Geometry: final body of the model. Coordinates: model frame, mm. Give positions to 0.01 mm unless a question says otherwise; leave off trailing zeros. Loops run counter-clockwise (first coordinate to the right, second up) from the corner with the lowest first, then second, coordinate; pieces in that order, holes last.
from build123d import *

# Parameters (mm, degrees)
SKETCH1_R           = 1.5875
BOSS_EXTRUDE5_DEPTH = 1.5875
FILLET2_R           = 2.54
FILLET3_R           = 2.54
FILLET4_R           = 5.08
CUT_EXTRUDE1_START  = -2.54
SKETCH2_R           = 2.38125
SKETCH2_R_2         = 1.5875
CUT_EXTRUDE1_DEPTH  = 2.54
SKETCH3_R           = 1.5875
CUT_EXTRUDE2_DEPTH  = 2.54
CUT_EXTRUDE3_DEPTH  = 2.54
SKETCH5_W           = 15
SKETCH5_H           = 34.925
CUT_EXTRUDE4_DEPTH  = 109.650407999
FILLET5_R           = 7.62
FILLET6_R           = 7.62
SKETCH6_R           = 79.375
CUT_EXTRUDE5_DEPTH  = 0.5875


with BuildPart() as part:
    # Sketch1 → Boss-Extrude5 (new body)
    with BuildSketch(Plane(origin=(0, 0, 0), x_dir=(1, 0, 0), z_dir=(0, 1, 0))):
        with BuildLine():
            ThreePointArc((-63.5, -47.625), (-35.497579143, -70.995158286), (0, -79.375))
            ThreePointArc((0, -79.375), (35.497579143, -70.995158286), (63.5, -47.625))
            Line((63.5, -47.625), (50.8, -47.625))
            Line((50.8, -47.625), (50.8, 22.225))
            Line((50.8, 22.225), (76.2, 22.225))
            ThreePointArc((76.2, 22.225), (0, 79.375), (-76.2, 22.225))
            Line((-76.2, 22.225), (-50.8, 22.225))
            Line((-50.8, 22.225), (-50.8, -47.625))
            Line((-50.8, -47.625), (-63.5, -47.625))
        make_face()
        with Locations(Location((-7.14375, -66.675, 0), (0, 0, 270))):
            Circle(SKETCH1_R, mode=Mode.SUBTRACT)
        with BuildLine():
            ThreePointArc((8.73125, -66.675), (7.14375, -68.2625), (5.55625, -66.675))
            ThreePointArc((5.55625, -66.675), (7.14375, -65.0875), (8.73125, -66.675))
        make_face(mode=Mode.SUBTRACT)
        with Locations(Location((-7.14375, 66.675, 0), (0, 0, 270))):
            Circle(SKETCH1_R, mode=Mode.SUBTRACT)
        with Locations(Location((7.14375, 66.675, 0), (0, 0, 270))):
            Circle(SKETCH1_R, mode=Mode.SUBTRACT)
    extrude(amount=BOSS_EXTRUDE5_DEPTH)

    # Fillet2
    fillet2_edges = [part.edges().sort_by_distance(p)[0] for p in [
        (-63.5, 0.79375, 47.625),
    ]]
    fillet(fillet2_edges, radius=FILLET2_R)

    # Fillet3
    fillet3_edges = [part.edges().sort_by_distance(p)[0] for p in [
        (63.5, 0.79375, 47.625),
    ]]
    fillet(fillet3_edges, radius=FILLET3_R)

    # Fillet4
    fillet4_edges = [part.edges().sort_by_distance(p)[0] for p in [
        (-76.2, 0.79375, -22.225),
        (76.2, 0.79375, -22.225),
    ]]
    fillet(fillet4_edges, radius=FILLET4_R)

    # Sketch2 → Cut-Extrude1 (cut)
    # profile 1 of 10: a face of its own
    with BuildSketch(Plane(origin=(0, 1.5875, 0), x_dir=(1, 0, 0), z_dir=(0, 1, 0)).offset(CUT_EXTRUDE1_START)):
        with BuildLine():
            Line((-61.088622125, 27.654457796), (-59.642408406, 26.999765402))
            ThreePointArc((-59.642408406, 26.999765402), (-52.384826382, 39.268743005), (-42.643785254, 49.676068599))
            Line((-42.643785254, 49.676068599), (-43.677815048, 50.880617741))
            Line((-43.677815048, 50.880617741), (-44.711844841, 52.085166883))
            ThreePointArc((-44.711844841, 52.085166883), (-54.925289002, 41.173126022), (-62.534835843, 28.309150189))
            Line((-62.534835843, 28.309150189), (-61.088622125, 27.654457796))
        make_face()
    # profile 2 of 10: a face of its own
    with BuildSketch(Plane(origin=(0, 1.5875, 0), x_dir=(1, 0, 0), z_dir=(0, 1, 0)).offset(CUT_EXTRUDE1_START)):
        with BuildLine():
            Line((-39.077069744, 54.493774041), (-38.151958122, 53.203686937))
            ThreePointArc((-38.151958122, 53.203686937), (-25.732218917, 60.200142208), (-12.092567045, 64.342629994))
            Line((-12.092567045, 64.342629994), (-12.385788543, 65.902815048))
            Line((-12.385788543, 65.902815048), (-12.679010041, 67.463000102))
            ThreePointArc((-12.679010041, 67.463000102), (-26.980132574, 63.119617589), (-40.002181367, 55.783861145))
            Line((-40.002181367, 55.783861145), (-39.077069744, 54.493774041))
        make_face()
    # profile 3 of 10: a face of its own
    with BuildSketch(Plane(origin=(0, 1.5875, 0), x_dir=(1, 0, 0), z_dir=(0, 1, 0)).offset(CUT_EXTRUDE1_START)):
        with Locations(Location((-7.14375, 66.675, 0), (0, 0, 270))):
            Circle(SKETCH2_R)
        with Locations((-7.14375, 66.675)):
            Circle(SKETCH2_R_2, mode=Mode.SUBTRACT)
    # profile 4 of 10: a face of its own
    with BuildSketch(Plane(origin=(0, 1.5875, 0), x_dir=(1, 0, 0), z_dir=(0, 1, 0)).offset(CUT_EXTRUDE1_START)):
        with Locations(Location((7.14375, 66.675, 0), (0, 0, 270))):
            Circle(SKETCH2_R)
        with Locations((7.14375, 66.675)):
            Circle(SKETCH2_R_2, mode=Mode.SUBTRACT)
    # profile 5 of 10: a face of its own
    with BuildSketch(Plane(origin=(0, 1.5875, 0), x_dir=(1, 0, 0), z_dir=(0, 1, 0)).offset(CUT_EXTRUDE1_START)):
        with BuildLine():
            ThreePointArc((12.679010041, 67.463000102), (26.980132574, 63.119617589), (40.002181367, 55.783861145))
            Line((40.002181367, 55.783861145), (39.077069744, 54.493774041))
            Line((39.077069744, 54.493774041), (38.151958122, 53.203686937))
            ThreePointArc((38.151958122, 53.203686937), (25.732218917, 60.200142208), (12.092567045, 64.342629994))
            Line((12.092567045, 64.342629994), (12.385788543, 65.902815048))
            Line((12.385788543, 65.902815048), (12.679010041, 67.463000102))
        make_face()
    # profile 6 of 10: a face of its own
    with BuildSketch(Plane(origin=(0, 1.5875, 0), x_dir=(1, 0, 0), z_dir=(0, 1, 0)).offset(CUT_EXTRUDE1_START)):
        with BuildLine():
            ThreePointArc((44.711844841, 52.085166883), (54.925289002, 41.173126022), (62.534835843, 28.309150189))
            Line((62.534835843, 28.309150189), (59.642408406, 26.999765402))
            ThreePointArc((59.642408406, 26.999765402), (52.384826382, 39.268743005), (42.643785254, 49.676068599))
            Line((42.643785254, 49.676068599), (43.677815048, 50.880617741))
            Line((43.677815048, 50.880617741), (44.711844841, 52.085166883))
        make_face()
    # profile 7 of 10: a face of its own
    with BuildSketch(Plane(origin=(0, 1.5875, 0), x_dir=(1, 0, 0), z_dir=(0, 1, 0)).offset(CUT_EXTRUDE1_START)):
        with BuildLine():
            ThreePointArc((-12.679010041, -67.463000102), (-26.980132574, -63.119617589), (-40.002181367, -55.783861145))
            Line((-40.002181367, -55.783861145), (-39.077069744, -54.493774041))
            Line((-39.077069744, -54.493774041), (-38.151958122, -53.203686937))
            ThreePointArc((-38.151958122, -53.203686937), (-25.732218917, -60.200142208), (-12.092567045, -64.342629994))
            Line((-12.092567045, -64.342629994), (-12.385788543, -65.902815048))
            Line((-12.385788543, -65.902815048), (-12.679010041, -67.463000102))
        make_face()
    # profile 8 of 10: a face of its own
    with BuildSketch(Plane(origin=(0, 1.5875, 0), x_dir=(1, 0, 0), z_dir=(0, 1, 0)).offset(CUT_EXTRUDE1_START)):
        with Locations(Location((-7.14375, -66.675, 0), (0, 0, 270))):
            Circle(SKETCH2_R)
        with Locations((-7.14375, -66.675)):
            Circle(SKETCH2_R_2, mode=Mode.SUBTRACT)
    # profile 9 of 10: a face of its own
    with BuildSketch(Plane(origin=(0, 1.5875, 0), x_dir=(1, 0, 0), z_dir=(0, 1, 0)).offset(CUT_EXTRUDE1_START)):
        with Locations(Location((7.14375, -66.675, 0), (0, 0, 270))):
            Circle(SKETCH2_R)
        with Locations((7.14375, -66.675)):
            Circle(SKETCH2_R_2, mode=Mode.SUBTRACT)
    # profile 10 of 10: a face of its own
    with BuildSketch(Plane(origin=(0, 1.5875, 0), x_dir=(1, 0, 0), z_dir=(0, 1, 0)).offset(CUT_EXTRUDE1_START)):
        with BuildLine():
            ThreePointArc((12.092567045, -64.342629994), (25.732218917, -60.200142208), (38.151958122, -53.203686937))
            Line((38.151958122, -53.203686937), (39.077069744, -54.493774041))
            Line((39.077069744, -54.493774041), (40.002181367, -55.783861145))
            ThreePointArc((40.002181367, -55.783861145), (26.980132574, -63.119617589), (12.679010041, -67.463000102))
            Line((12.679010041, -67.463000102), (12.385788543, -65.902815048))
            Line((12.385788543, -65.902815048), (12.092567045, -64.342629994))
        make_face()
    extrude(amount=CUT_EXTRUDE1_DEPTH, mode=Mode.SUBTRACT)

    # Sketch3 → Cut-Extrude2 (cut)
    with BuildSketch(Plane(origin=(0, 1.5875, 0), x_dir=(1, 0, 0), z_dir=(0, 1, 0))):
        with Locations(Location((-44.45, -47.625, 0), (0, 0, 270))):
            Circle(SKETCH3_R)
        with Locations(Location((-44.45, 22.225, 0), (0, 0, 270))):
            Circle(SKETCH3_R)
        with Locations(Location((44.45, 22.225, 0), (0, 0, 270))):
            Circle(SKETCH3_R)
        with Locations(Location((44.45, -47.625, 0), (0, 0, 270))):
            Circle(SKETCH3_R)
    extrude(amount=-CUT_EXTRUDE2_DEPTH, mode=Mode.SUBTRACT)

    # Sketch4 → Cut-Extrude3 (cut)
    with BuildSketch(Plane(origin=(0, 1.5875, 0), x_dir=(1, 0, 0), z_dir=(0, 1, 0))):
        with BuildLine():
            ThreePointArc((-44.45, -11.1125), (-46.0375, -12.7), (-44.45, -14.2875))
            Line((-44.45, -14.2875), (-44.45, -11.1125))
        make_face()
        with BuildLine():
            Line((-44.45, -11.1125), (-44.45, -14.2875))
            ThreePointArc((-44.45, -14.2875), (-43.327467985, -13.822532015), (-42.8625, -12.7))
            ThreePointArc((-42.8625, -12.7), (-43.327467985, -11.577467985), (-44.45, -11.1125))
        make_face()
        with BuildLine():
            ThreePointArc((44.45, -11.1125), (42.8625, -12.7), (44.45, -14.2875))
            Line((44.45, -14.2875), (44.45, -11.1125))
        make_face()
        with BuildLine():
            Line((44.45, -11.1125), (44.45, -14.2875))
            ThreePointArc((44.45, -14.2875), (45.572532015, -13.822532015), (46.0375, -12.7))
            ThreePointArc((46.0375, -12.7), (45.572532015, -11.577467985), (44.45, -11.1125))
        make_face()
    extrude(amount=-CUT_EXTRUDE3_DEPTH, mode=Mode.SUBTRACT)

    # Sketch5 → Cut-Extrude4 (cut, through all)
    with BuildSketch(Plane(origin=(0, 1.5875, 0), x_dir=(1, 0, 0), z_dir=(0, 1, 0))):
        with Locations((-27.3, 4.7625)):
            Rectangle(SKETCH5_W, SKETCH5_H)
        with Locations((27.3, 4.7625)):
            Rectangle(SKETCH5_W, SKETCH5_H)
    extrude(amount=-CUT_EXTRUDE4_DEPTH, mode=Mode.SUBTRACT)

    # Fillet5
    # the kernel refuses this fillet: 7.62 mm, written as the material it adds along each edge
    with BuildSketch(Plane(origin=(-19.8, 1.5875, 12.7), x_dir=(0, 0, -1), z_dir=(0, -1, 0))) as fillet5_piece_1:
        with BuildLine():
            CenterArc((FILLET5_R, -FILLET5_R), FILLET5_R, 90, 90)
            Line((0, -FILLET5_R), (0, 0))
            Line((0, 0), (FILLET5_R, 0))
        make_face()
    extrude(amount=1.5875)
    with BuildSketch(Plane(origin=(-34.8, 1.5875, 12.7), x_dir=(0, 0, -1), z_dir=(0, -1, 0)), Plane(origin=(-19.8, 1.5875, -22.225), x_dir=(0, 0, 1), z_dir=(0, -1, 0)), Plane(origin=(-34.8, 1.5875, -22.225), x_dir=(1, 0, 0), z_dir=(0, -1, 0))) as fillet5_piece_2:
        with BuildLine():
            CenterArc((FILLET5_R, FILLET5_R), FILLET5_R, 180, 90)
            Line((0, FILLET5_R), (0, 0))
            Line((0, 0), (FILLET5_R, 0))
        make_face()
    extrude(amount=1.5875)

    # Fillet6
    # the kernel refuses this fillet: 7.62 mm, written as the material it adds along each edge
    with BuildSketch(Plane(origin=(34.8, 1.5875, 12.7), x_dir=(0, 0, -1), z_dir=(0, -1, 0)), Plane(origin=(34.8, 1.5875, -22.225), x_dir=(-1, 0, 0), z_dir=(0, -1, 0))) as fillet6_piece_1:
        with BuildLine():
            CenterArc((FILLET6_R, -FILLET6_R), FILLET6_R, 90, 90)
            Line((0, -FILLET6_R), (0, 0))
            Line((0, 0), (FILLET6_R, 0))
        make_face()
    extrude(amount=1.5875)
    with BuildSketch(Plane(origin=(19.8, 1.5875, -22.225), x_dir=(1, 0, 0), z_dir=(0, -1, 0)), Plane(origin=(19.8, 1.5875, 12.7), x_dir=(0, 0, -1), z_dir=(0, -1, 0))) as fillet6_piece_2:
        with BuildLine():
            CenterArc((FILLET6_R, FILLET6_R), FILLET6_R, 180, 90)
            Line((0, FILLET6_R), (0, 0))
            Line((0, 0), (FILLET6_R, 0))
        make_face()
    extrude(amount=1.5875)

    # Sketch6 → Cut-Extrude5 (cut)
    with BuildSketch(Plane(origin=(0, 0, 0), x_dir=(-1, 0, 0), z_dir=(0, -1, 0))):
        Circle(SKETCH6_R)
    extrude(amount=-CUT_EXTRUDE5_DEPTH, mode=Mode.SUBTRACT)


solid = part.part
Item 1: Section query C-C on z = 32. Return loops of the section in (x, y).
Values follow:
outline: (-50.8, 0.59) - (50.8, 0.59) - (50.8, 1.59) - (-50.8, 1.59) - close
Item 2: Pin query (flat end, axial travel): pin 1 (0.5 mm diameter, centred on y = 1, z = -6.5, fed in from +X); pin 2 (1.9 mm diameter, centred on x = 44.45, z = -22.225, fed in from +Y); pin 3 (0.5 mm diameter, centred on x = -54, y = 1, fed in from -Z). Return the tip coordinate at first contact, or that it passes through.
Values follow:
pin 1: stops at x = 50.8
pin 2: passes through
pin 3: stops at z = -58.41
Item 3: Section query D-D on y = 1.2. Give the number of separate pieces and of enclosed holes in the cut face, plus the area to 3 significant figures.
Values follow:
separate pieces: 1
enclosed holes: 18
area: 14,700 mm2
Item 4: Ray query, probe 1 along X at (y, z) = (1.15, -13); probe 2 along Z at (x, y) = (52.5, 1.3) (3 decimals); probe 3 along Z at (x, y) = (37, 1). Return the intervals inside material, ascending.
Values follow:
probe 1: x = -50.8 to -34.8, -19.8 to 19.8, 34.8 to 50.8
probe 2: z = -59.533 to -44.224, -39.115 to -22.225, 47.625 to 59.533
probe 3: z = -70.22 to -57.82, -54.01 to 54.01, 57.82 to 70.22
Item 5: Section query A-A on x = -22.5. Return loops of the section in (y, z).
Values follow:
outline: (0.59, -76.12) - (1.59, -76.12) - (1.59, -64.85) - (0.59, -64.85) - close; (0.59, -61.48) - (1.59, -61.48) - (1.59, -20.42) - (0.59, -20.42) - close; (0.59, 10.9) - (1.59, 10.9) - (1.59, 61.48) - (0.59, 61.48) - close; (0.59, 64.85) - (1.59, 64.85) - (1.59, 76.12) - (0.59, 76.12) - close
Item 6: Section query B-B on x = 25.5. Return loops of the section in (y, z), plus the area to 3 significant figures.
Values follow:
outline: (0.59, -75.17) - (1.59, -75.17) - (1.59, -63.73) - (0.59, -63.73) - close; (0.59, -60.3) - (1.59, -60.3) - (1.59, -21.98) - (0.59, -21.98) - close; (0.59, 12.45) - (1.59, 12.45) - (1.59, 60.3) - (0.59, 60.3) - close; (0.59, 63.73) - (1.59, 63.73) - (1.59, 75.17) - (0.59, 75.17) - close
area: 109 mm2
